from build123d import *

# Parameters (mm, degrees)
SALIENTE_EXTRUIR1_DEPTH = 60
CROQUIS2_W              = 5
CROQUIS2_H              = 41
CORTAR_EXTRUIR1_DEPTH   = 20
CROQUIS4_R              = 10.5
CORTAR_EXTRUIR3_DEPTH   = 1.5
CROQUIS5_R              = 5
CORTAR_EXTRUIR4_DEPTH   = 51.5
CROQUIS7_R              = 2.2
CROQUIS7_R_2            = 2.253524607
CORTAR_EXTRUIR5_DEPTH   = 10
CROQUIS8_R              = 1.5
CORTAR_EXTRUIR6_DEPTH   = 10
CORTAR_EXTRUIR7_DEPTH   = 3


with BuildPart() as part:
    # Croquis1 → Saliente-Extruir1 (new body)
    with BuildSketch(Plane.XY):
        Polygon((0, 0), (40, 0), (40, 5), (31, 5), (31, 25), (26, 25), (26, 5), (5, 5), (5, 30), (0, 30), align=None)
    extrude(amount=SALIENTE_EXTRUIR1_DEPTH)

    # Croquis2 → Cortar-Extruir1 (cut)
    with BuildSketch(Plane(origin=(0, 25, 0), x_dir=(1, 0, 0), z_dir=(0, 1, 0))):
        with Locations((28.5, -30)):
            Rectangle(CROQUIS2_W, CROQUIS2_H)
    extrude(amount=-CORTAR_EXTRUIR1_DEPTH, mode=Mode.SUBTRACT)

    # Croquis4 → Cortar-Extruir3 (cut)
    with BuildSketch(Plane.XZ):
        with Locations(Location((20, 35, 0), (0, 0, 270))):
            Circle(CROQUIS4_R)
    extrude(amount=-CORTAR_EXTRUIR3_DEPTH, mode=Mode.SUBTRACT)

    # Croquis5 → Cortar-Extruir4 (cut)
    with BuildSketch(Plane.XZ.offset(-1.5)):
        with Locations(Location((20, 35, 0), (0, 0, 270))):
            Circle(CROQUIS5_R)
    extrude(amount=-CORTAR_EXTRUIR4_DEPTH, mode=Mode.SUBTRACT)

    # Croquis7 → Cortar-Extruir5 (cut)
    with BuildSketch(Plane(origin=(31, 0, 0), x_dir=(0, 0, -1), z_dir=(1, 0, 0))):
        with Locations(Location((-53.9, 20.1, 0), (0, 0, 90))):
            Circle(CROQUIS7_R)
        with Locations(Location((-53.9, 9.9, 0), (0, 0, 90))):
            Circle(CROQUIS7_R)
        with Locations(Location((-6.1, 9.9, 0), (0, 0, 90))):
            Circle(CROQUIS7_R)
        with Locations(Location((-6.1, 20.1, 0), (0, 0, 90))):
            Circle(CROQUIS7_R_2)
    extrude(amount=-CORTAR_EXTRUIR5_DEPTH, mode=Mode.SUBTRACT)

    # Croquis8 → Cortar-Extruir6 (cut)
    with BuildSketch(Plane.ZY):
        with Locations(Location((20, 15, 0), (0, 0, 270))):
            Circle(CROQUIS8_R)
    extrude(amount=-CORTAR_EXTRUIR6_DEPTH, mode=Mode.SUBTRACT)

    # Croquis9 → Cortar-Extruir7 (cut)
    with BuildSketch(Plane(origin=(5, 0, 0), x_dir=(0, 0, -1), z_dir=(1, 0, 0))):
        Polygon((-18.435990885, 18.090934404), (-21.894823157, 17.899938827), (-23.458832273, 14.809004424), (-21.564009115, 11.909065596), (-18.105176843, 12.100061173), (-16.541167727, 15.190995576), align=None)
    extrude(amount=-CORTAR_EXTRUIR7_DEPTH, mode=Mode.SUBTRACT)


solid = part.part
Part model, mm, in its own coordinate system. A direction names the side the tool comes from. Coordinates: 2 decimals unless noted, no trailing zeros. Write each loop counter-clockwise with the first axis right and the second up, starting at its lowest first coordinate (ties: lowest second). Pieces come first, ordered by that corner, then holes. Notation, with made-up numbers: M 42,23.25 L 78,23.25 A24 ccw 78,35.25 Z; hole C 82.5,61 d2. An arc over 180 degrees is marked long. Return JSON: item names as keys, results as strings.
1. 3-axis set-ups, long thin cutter, end or side, ignore diameter. For faces 3 (the face through (3.521, 16.376, 22.666)), 4 (the face through (18, 1.5, 30)), 5 (the face through (26, 15, 5)), 6 (the face through (28, 15, 9.5)): which of +Z, -Z, +X, -X, +Y, -Y reach the whole face in a straight line?
Determined:
{"face 3": "+X", "face 4": "-Y", "face 5": "+Z, -Z, +Y", "face 6": "+X, +Y"}
2. Pull direction Z, two halves, no side cores. Call faces 1 (the face through (31, 15, 5)), 2 (the face through (0.99, 16.11, 21.01)): pulls with the +Z half, pulls with the -Z half, needs draft (parallel to the pull), parting line crosses it, or undercut.
Determined:
{"face 1": "needs draft", "face 2": "undercut"}
3. Saw through at C-C, the plane x = 20. Write the cut outline in (y, z).
Determined:
{"outline": "M 0,0 L 5,0 L 5,30 L 1.5,30 L 1.5,24.5 L 0,24.5 Z; M 0,45.5 L 1.5,45.5 L 1.5,40 L 5,40 L 5,60 L 0,60 Z"}
4. Probe L1, parallel to Z at x = 29, y = 20.1; L2, parallel to Z at x = 27.4, y = 9.9; L3, parallel to Z at x = 1.25, y = 15. List the from-to ranges inside material, lowest first.
Determined:
{"L1": "0 to 3.85, 8.35 to 9.5, 50.5 to 51.7, 56.1 to 60", "L2": "0 to 3.9, 8.3 to 9.5, 50.5 to 51.7, 56.1 to 60", "L3": "0 to 18.5, 21.5 to 60"}
5. Saw through at B-B, the plane y = 20.1. Write the cut outline in (x, z).
Determined:
{"outline": "M 0,0 L 5,0 L 5,60 L 0,60 Z; M 26,0 L 31,0 L 31,3.85 L 26,3.85 Z; M 26,8.35 L 31,8.35 L 31,9.5 L 26,9.5 Z; M 26,50.5 L 31,50.5 L 31,51.7 L 26,51.7 Z; M 26,56.1 L 31,56.1 L 31,60 L 26,60 Z"}
6. Flat gauge pins, fed straight in: pin 1 Ø1 at (y, z) = (17.5, 40) entering from +X; pin 2 Ø4 at (x, z) = (29.5, 57) entering from +Y; pin 3 Ø7.5 at (y, z) = (15.5, 4) entering from +X. Where does each tip first touch, or does it go through?
Determined:
{"pin 1": "x = 5", "pin 2": "y = 25", "pin 3": "x = 31"}
7. Saw through at A-A, the plane z = 53.9. Write the cut outline in (x, y), then the cut area to 3 significant figures.
Determined:
{"outline": "M 0,0 L 40,0 L 40,5 L 31,5 L 31,7.7 L 26,7.7 L 26,5 L 5,5 L 5,30 L 0,30 Z; M 26,12.1 L 31,12.1 L 31,17.9 L 26,17.9 Z; M 26,22.3 L 31,22.3 L 31,25 L 26,25 Z", "area": "381 mm²"}
8. Saw through at D-D, the plane z = 35. Write the cut outline in (x, y).
Determined:
{"outline": "M 0,0 L 9.5,0 L 9.5,1.5 L 15,1.5 L 15,5 L 5,5 L 5,30 L 0,30 Z; M 25,1.5 L 30.5,1.5 L 30.5,0 L 40,0 L 40,5 L 25,5 Z"}
